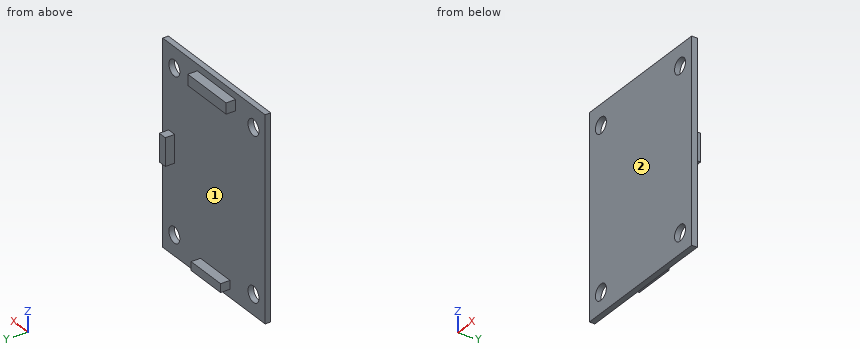
```python
from build123d import *

# Parameters (mm, degrees)
SKETCH1_W           = 31.518490379
SKETCH1_H           = 42.979759609
SKETCH1_R           = 1.685
BOSS_EXTRUDE1_DEPTH = 1.2
SKETCH2_W           = 9.074610473
SKETCH2_H           = 1.814922095
SKETCH2_W_2         = 1.853537458
SKETCH2_H_2         = 5.908150648
SKETCH2_W_3         = 11.777685933
SKETCH2_H_3         = 2.316921823
BOSS_EXTRUDE2_DEPTH = 2


with BuildPart() as part:
    # Sketch1 → Boss-Extrude1 (new body)
    with BuildSketch(Plane(origin=(0, 0, 0), x_dir=(1, 0, 0), z_dir=(0, 1, 0))):
        with Locations((12.186773079, 17.109376158)):
            Rectangle(SKETCH1_W, SKETCH1_H)
        with Locations(Location((0, 0, 0), (0, 0, 270))):
            Circle(SKETCH1_R, mode=Mode.SUBTRACT)
        with Locations(Location((24.37, 0, 0), (0, 0, 270))):
            Circle(SKETCH1_R, mode=Mode.SUBTRACT)
        with Locations(Location((24.37, 34.27, 0), (0, 0, 270))):
            Circle(SKETCH1_R, mode=Mode.SUBTRACT)
        with Locations(Location((0, 34.27, 0), (0, 0, 270))):
            Circle(SKETCH1_R, mode=Mode.SUBTRACT)
    extrude(amount=BOSS_EXTRUDE1_DEPTH)

    # Sketch2 → Boss-Extrude2 (add)
    with BuildSketch(Plane(origin=(0, 1.2, 0), x_dir=(1, 0, 0), z_dir=(0, 1, 0))):
        with Locations((11.781311759, 35.95367365)):
            Rectangle(SKETCH2_W, SKETCH2_H)
        with Locations((25.20015065, 16.530145702)):
            Rectangle(SKETCH2_W_2, SKETCH2_H_2)
        with Locations((11.433773487, -1.792844381)):
            Rectangle(SKETCH2_W_3, SKETCH2_H_3)
    extrude(amount=BOSS_EXTRUDE2_DEPTH)


solid = part.part
```
Input: part model. Units: mm. Frame: model coordinates. Face numbers are marked on the shaded views. Coordinates: 2 decimals unless noted, no trailing zeros. Write each loop counter-clockwise with the first axis right and the second up, starting at its lowest first coordinate (ties: lowest second). Pieces come first, ordered by that corner, then holes.
1) Section B-B on z = -34.27. Output: boundary loops of the cut face in (x, y) (3 decimals), and give its area (3 significant figures).
2) Section D-D on x = 11. Output: boundary loops of the cut face in (y, z), and give its area (3 significant figures).
3) Mould query, pull axis Z, two halves, no side actions, for the marked faces 1 and 2. Classes: pulls with the +Z half, pulls with the -Z half, needs draft (parallel to the pull), parting line crosses it, or undercut.
4) Section C-C on y = 0.5. Output: boundary loops of the cut face in (x, z) (1 decimal).
5) Material intervals for line 1 along X through (y, z) = (0.8, -34.27) (3 decimals); line 2 along Z through (x, y) = (15.5, 2.6); line 3 along Y through (x, z) = (-0.5, -25), sorted ascending.
6) Pin query (flat end, axial travel): pin 1 Ø0.6 at (x, y) = (13, 2.5) entering from -Z; pin 2 Ø1.6 at (x, y) = (12, 2.5) entering from +Z; pin 3 Ø1 at (y, z) = (2, -16.5) entering from +X; pin 4 Ø1 at (x, z) = (1, -9) entering from -Y. Return the tip coordinate at first contact, or that it passes through.
7) Section A-A on x = 0. Output: boundary loops of the cut face in (y, z) (1 decimal), and give its area (3 significant figures).
Check result:
1. outline: (-3.572, 0) - (-1.685, 0) - (-1.685, 1.2) - (-3.572, 1.2) - close; (1.685, 0) - (22.685, 0) - (22.685, 1.2) - (1.685, 1.2) - close; (26.055, 0) - (27.946, 0) - (27.946, 1.2) - (26.055, 1.2) - close
1. area: 29.7 mm2
2. outline: (0, -38.6) - (1.2, -38.6) - (1.2, -36.86) - (3.2, -36.86) - (3.2, -35.05) - (1.2, -35.05) - (1.2, 0.63) - (3.2, 0.63) - (3.2, 2.95) - (1.2, 2.95) - (1.2, 4.38) - (0, 4.38) - close
2. area: 59.8 mm2
3. face 1: undercut
3. face 2: needs draft
4. outline: (-3.6, -38.6) - (27.9, -38.6) - (27.9, 4.4) - (-3.6, 4.4) - close; hole circle Ø3.4 at (0, -34.3); hole circle Ø3.4 at (0, 0); hole circle Ø3.4 at (24.4, -34.3); hole circle Ø3.4 at (24.4, 0)
5. line 1: x = -3.572 to -1.685, 1.685 to 22.685, 26.055 to 27.946
5. line 2: z = -36.86 to -35.05, 0.63 to 2.95
5. line 3: y = 0 to 1.2
6. pin 1: stops at z = -36.86
6. pin 2: stops at z = 2.95
6. pin 3: stops at x = 26.13
6. pin 4: stops at y = 0
7. outline: (0, -38.6) - (1.2, -38.6) - (1.2, -36) - (0, -36) - close; (0, -32.6) - (1.2, -32.6) - (1.2, -1.7) - (0, -1.7) - close; (0, 1.7) - (1.2, 1.7) - (1.2, 4.4) - (0, 4.4) - close
7. area: 43.5 mm2
